from build123d import *

# Parameters (mm, degrees)
BOSS_EXTRUDE2_DEPTH = 25.4
CUT_EXTRUDE1_REACH  = 41.741
SKETCH4_R           = 1.55
RIB12_REACH         = 41.741
SKETCH8_WALL_W      = 105.149018068
SKETCH8_WALL_H      = 5
CUT_EXTRUDE2_REACH  = 39.872
SKETCH5_R           = 1.55


with BuildPart() as part:
    # Sketch3 → Boss-Extrude2 (new body)
    with BuildSketch(Plane(origin=(0, 0, 0), x_dir=(0, 0, -1), z_dir=(1, 0, 0))):
        Polygon((0, 0), (0, 5), (20.4, 5), (20.4, 17), (25.4, 17), (25.4, 0), align=None)
    extrude(amount=BOSS_EXTRUDE2_DEPTH)

    # Sketch4 → Cut-Extrude1 (cut, up to next)
    with BuildSketch(Plane(origin=(0, 0, -25.4), x_dir=(-1, 0, 0), z_dir=(0, 0, -1)), mode=Mode.PRIVATE) as cut_extrude1_sk1:
        with Locations(Location((-16.2, 12, 0), (0, 0, 90))):
            Circle(SKETCH4_R)
    cut_extrude1_tool1 = extrude(cut_extrude1_sk1.sketch, amount=-CUT_EXTRUDE1_REACH, mode=Mode.PRIVATE) & part.part
    # Sketch4 → Cut-Extrude1 (cut, up to next)
    with BuildSketch(Plane(origin=(0, 0, -25.4), x_dir=(-1, 0, 0), z_dir=(0, 0, -1)), mode=Mode.PRIVATE) as cut_extrude1_sk2:
        with Locations(Location((-9.2, 12, 0), (0, 0, 90))):
            Circle(SKETCH4_R)
    cut_extrude1_tool2 = extrude(cut_extrude1_sk2.sketch, amount=-CUT_EXTRUDE1_REACH, mode=Mode.PRIVATE) & part.part
    add(cut_extrude1_tool1.solids().sort_by_distance((16.2, 12, -25.4))[0], mode=Mode.SUBTRACT)
    add(cut_extrude1_tool2.solids().sort_by_distance((9.2, 12, -25.4))[0], mode=Mode.SUBTRACT)

    # Sketch8 wall → Rib12 (add, up to next)
    with BuildSketch(Plane(origin=(0, 11, -10.2), x_dir=(0, -0.507020126563, 0.861934215158), z_dir=(0, 0.861934215158, 0.507020126563)), mode=Mode.PRIVATE) as rib12_sk1:
        with Locations((0, 2.5)):
            Rectangle(SKETCH8_WALL_W, SKETCH8_WALL_H)
    rib12_tool1 = extrude(rib12_sk1.sketch, amount=-RIB12_REACH, mode=Mode.PRIVATE) - part.part
    rib12 = rib12_tool1.solids().sort_by_distance((0, 11, -10.2))[0]
    add(rib12)

    # Mirror1: Rib12 across plane
    add(rib12.mirror(Plane(origin=(12.7, 0, 0), x_dir=(0, 0, 1), z_dir=(1, 0, 0))))

    # Sketch5 → Cut-Extrude2 (cut, up to next)
    with BuildSketch(Plane(origin=(0, 5, 0), x_dir=(1, 0, 0), z_dir=(0, 1, 0)), mode=Mode.PRIVATE) as cut_extrude2_sk1:
        with Locations(Location((9, 4, 0), (0, 0, 270))):
            Circle(SKETCH5_R)
    cut_extrude2_tool1 = extrude(cut_extrude2_sk1.sketch, amount=-CUT_EXTRUDE2_REACH, mode=Mode.PRIVATE) & part.part
    # Sketch5 → Cut-Extrude2 (cut, up to next)
    with BuildSketch(Plane(origin=(0, 5, 0), x_dir=(1, 0, 0), z_dir=(0, 1, 0)), mode=Mode.PRIVATE) as cut_extrude2_sk2:
        with Locations(Location((9, 13.4, 0), (0, 0, 270))):
            Circle(SKETCH5_R)
    cut_extrude2_tool2 = extrude(cut_extrude2_sk2.sketch, amount=-CUT_EXTRUDE2_REACH, mode=Mode.PRIVATE) & part.part
    # Sketch5 → Cut-Extrude2 (cut, up to next)
    with BuildSketch(Plane(origin=(0, 5, 0), x_dir=(1, 0, 0), z_dir=(0, 1, 0)), mode=Mode.PRIVATE) as cut_extrude2_sk3:
        with Locations(Location((16.4, 13.4, 0), (0, 0, 270))):
            Circle(SKETCH5_R)
    cut_extrude2_tool3 = extrude(cut_extrude2_sk3.sketch, amount=-CUT_EXTRUDE2_REACH, mode=Mode.PRIVATE) & part.part
    # Sketch5 → Cut-Extrude2 (cut, up to next)
    with BuildSketch(Plane(origin=(0, 5, 0), x_dir=(1, 0, 0), z_dir=(0, 1, 0)), mode=Mode.PRIVATE) as cut_extrude2_sk4:
        with Locations(Location((16.4, 4, 0), (0, 0, 270))):
            Circle(SKETCH5_R)
    cut_extrude2_tool4 = extrude(cut_extrude2_sk4.sketch, amount=-CUT_EXTRUDE2_REACH, mode=Mode.PRIVATE) & part.part
    add(cut_extrude2_tool1.solids().sort_by_distance((9, 5, -4))[0], mode=Mode.SUBTRACT)
    add(cut_extrude2_tool2.solids().sort_by_distance((9, 5, -13.4))[0], mode=Mode.SUBTRACT)
    add(cut_extrude2_tool3.solids().sort_by_distance((16.4, 5, -13.4))[0], mode=Mode.SUBTRACT)
    add(cut_extrude2_tool4.solids().sort_by_distance((16.4, 5, -4))[0], mode=Mode.SUBTRACT)


solid = part.part
Check sheet for the modelled part. Datum: model origin and axes. Units: mm. A direction names the side the tool comes from. Round coordinates to 2 decimals unless told otherwise and drop trailing zeros. Loops run counter-clockwise (first coordinate to the right, second up) from the corner with the lowest first, then second, coordinate; pieces in that order, holes last. Notation, with made-up numbers: M -35.75,-7 L -3.75,-7 A9 ccw -3.75,9 Z; hole C 59.25,-24.75 d3. An arc over 180 degrees is marked long. One line per item, written item: value.
(1) Sectioned sample at D-D, the plane x = 8.5. Record the cut outline in (y, z).
Computed values:
outline: M 0,-25.4 L 10.62,-25.4 L 10.62,-20.4 L 5,-20.4 L 5,-14.87 L 0,-14.87 Z; M 0,-11.93 L 5,-11.93 L 5,-5.47 L 0,-5.47 Z; M 0,-2.53 L 5,-2.53 L 5,0 L 0,0 Z; M 13.38,-25.4 L 17,-25.4 L 17,-20.4 L 13.38,-20.4 Z
(2) Depth check by flat-ended pin: pin 1 Ø6 at (x, y) = (15.5, 9.5) entering from +Z; pin 2 Ø2.5 at (x, z) = (16.4, -4) entering from -Y; pin 3 Ø6 at (x, z) = (11.5, -7.5) entering from +Y; pin 4 Ø3 at (x, z) = (20.5, -16.5) entering from +Y. Enter the tip coordinate at first touch or a pass-through.
Computed values:
pin 1: stops at z = -20.4
pin 2: passes through
pin 3: stops at y = 5
pin 4: stops at y = 15.59
(3) Access from +Z, -Z, +X, -X, +Y, -Y to the whole of each face (thin tool, end or side, straight path). Record for faces 1 (the face through (14.887, 2.535, -4.336)), 2 (the face through (20.4, 9, -15)).
Computed values:
face 1: +Y, -Y
face 2: +Z, +Y
(4) Thickness scan on line 1 (X direction, y = 6, z = -8.5); line 2 (Y direction, x = 11.75, z = -4.5); line 3 (Z direction, x = 15.5, y = 4.25). Record the ranges inside material, lowest first.
Computed values:
line 1: x = 0 to 5, 20.4 to 25.4
line 2: y = 0 to 5
line 3: z = -25.4 to -14.66, -12.14 to -5.26, -2.74 to 0
(5) Sectioned sample at C-C, the plane z = -3.75. Record the cut outline in (x, y), then the cut area to 3 significant figures.
Computed values:
outline: M 0,0 L 7.47,0 L 7.47,5 L 5,5 L 5,7.21 L 0,7.21 Z; M 10.53,0 L 14.87,0 L 14.87,5 L 10.53,5 Z; M 17.93,0 L 25.4,0 L 25.4,7.21 L 20.4,7.21 L 20.4,5 L 17.93,5 Z
area: 118 mm^2
(6) Sectioned sample at B-B, the plane y = 1.5. Record the cut outline in (x, z).
Computed values:
outline: M 0,-25.4 L 25.4,-25.4 L 25.4,0 L 0,0 Z; hole C 9,-13.4 d3.1; hole C 9,-4 d3.1; hole C 16.4,-13.4 d3.1; hole C 16.4,-4 d3.1
(7) Release check for a two-part mould opening along Z. For faces 3 (the face through (22.865, 11.084, -10.343)), 4 (the face through (8.06, 2.54, -5.23)), 5 (the face through (9.466, 2.535, -11.922)), 6 (the face through (25.4, 6, -14)) record: +Z half, -Z half, draft (parallel to the pull), parting line (faces both ways), or undercut.
Computed values:
face 3: +Z half
face 4: undercut
face 5: undercut
face 6: draft
(8) Sectioned sample at A-A, the plane y = 12. Record the cut outline in (x, z), then the cut area to 3 significant figures.
Computed values:
outline: M 0,-25.4 L 7.65,-25.4 L 7.65,-20.4 L 5,-20.4 L 5,-11.9 L 0,-11.9 Z; M 10.75,-25.4 L 14.65,-25.4 L 14.65,-20.4 L 10.75,-20.4 Z; M 17.75,-25.4 L 25.4,-25.4 L 25.4,-11.9 L 20.4,-11.9 L 20.4,-20.4 L 17.75,-20.4 Z
area: 181 mm^2
